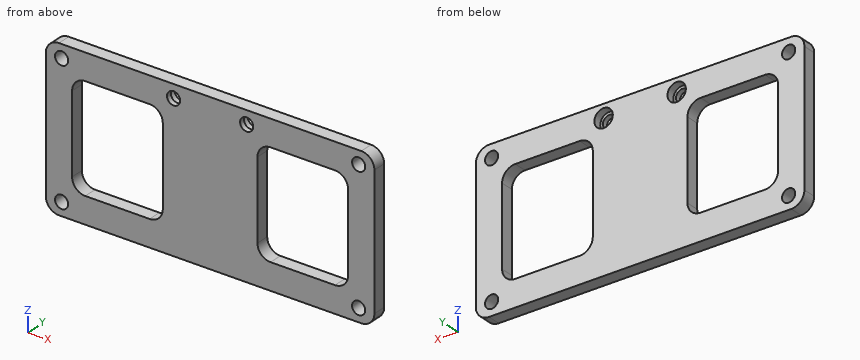
Autodesk Inventor part; units mm, degrees
ref_plane "YZ Plane" through (0, 0, 0) normal (1, 0, 0) x (0, 1, 0)
ref_plane "XZ Plane" through (0, 0, 0) normal (0, 1, 0) x (-1, 0, 0)
ref_plane "XY Plane" through (0, 0, 0) normal (0, 0, 1) x (1, 0, 0)
sketch "Sketch1" plane through (0, 0, 0) normal (0, 1, 0) x (-1, 0, 0)
  line L0 (33.3375, 19.05) -> (-33.3375, 19.05)
  line L1 (-33.3375, 19.05) -> (-33.3375, -19.05)
  line L2 (-33.3375, -19.05) -> (33.3375, -19.05)
  line L3 (33.3375, -19.05) -> (33.3375, 19.05)
  line L4 (33.3375, 19.05) -> (-33.3375, -19.05) construction
  line L5 (-33.3375, 19.05) -> (33.3375, -19.05) construction
  line L6 (39.6875, -19.05) -> (-39.6875, -19.05)
  line L7 (-39.6875, -19.05) -> (-39.6875, 19.05)
  line L8 (-39.6875, 19.05) -> (39.6875, 19.05)
  line L9 (39.6875, 19.05) -> (39.6875, -19.05)
  line L10 (39.6875, -19.05) -> (-39.6875, 19.05) construction
  line L11 (-39.6875, -19.05) -> (39.6875, 19.05) construction
  circle A0 centre (35.8775, -15.875) radius 1.5875
  circle A1 centre (35.8775, 15.875) radius 1.5875
  circle A2 centre (-35.8775, -15.875) radius 1.5875
  circle A3 centre (-35.8775, 15.875) radius 1.5875
  line L12 (33.3375, 12.7) -> (-33.3375, 12.7)
  line L13 (-33.3375, 12.7) -> (-33.3375, -12.7)
  line L14 (-33.3375, -12.7) -> (33.3375, -12.7)
  line L15 (33.3375, -12.7) -> (33.3375, 12.7)
  line L16 (11.43, 12.7) -> (-11.43, 12.7)
  line L17 (-11.43, 12.7) -> (-11.43, -12.7)
  line L18 (-11.43, -12.7) -> (11.43, -12.7)
  line L19 (11.43, -12.7) -> (11.43, 12.7)
  circle A4 centre (8.8265, 15.875) radius 1.5875
  circle A5 centre (-8.8265, 15.875) radius 1.5875
  point P0 (0, 0)
  point P1 (0, 12.7)
  point P2 (0, 0)
  point P3 (0, 0)
  point P4 (0, -12.7)
  point P5 (0, 0)
  point P6 (-11.43, -12.7)
  point P7 (-11.43, 12.7)
  point P8 (11.43, -12.7)
  point P9 (11.43, 12.7)
  dimension "d0" = 66.675
  dimension "d1" = 38.1
  dimension "d2" = 6.35
  dimension "d5" = 31.75
  dimension "d8" = 71.755
  dimension "d11" = 2.54
  dimension "d12" = 3.175
  dimension "d14" = 3.175
  dimension "d15" = 66.675
  dimension "d19" = 22.86
  dimension "d23" = 3.175
  dimension "d24" = 3.175
  dimension "d25" = 17.653
  dimension "d26" = 8.8265
  dimension "d28" = 6.35
  dimension "d29" = 6.35
extrude "Extrusion1" add sketch "Sketch1" along normal blind 3.175 contours L3 L12 L1 L0 | L8 L9 L6 L3 | L1 L6 L7 L8 | L3 L2 L1 L14 | L19 L14 L17 L12
fillet "Fillet1" radius 3.175 12 edges at (-39.6875, 1.5875, 19.05) (39.6875, 1.5875, 19.05) (-39.6875, 1.5875, -19.05) (39.6875, 1.5875, -19.05) (-33.3375, 1.5875, 12.7) (11.43, 1.5875, 12.7) (33.3375, 1.5875, 12.7) (11.43, 1.5875, -12.7) (33.3375, 1.5875, -12.7) (-11.43, 1.5875, -12.7) (-33.3375, 1.5875, -12.7) (-11.43, 1.5875, 12.7)
sketch "Sketch3" plane through (0, 3.175, 0) normal (0, 1, 0) x (1, 0, 0)
  circle A0 centre (-8.8265, -15.875) radius 1.5875
  circle A1 centre (-8.8265, -15.875) radius 2.2225
  circle A2 centre (8.8265, -15.875) radius 1.5875
  circle A3 centre (8.8265, -15.875) radius 2.2225
  point P0 (0, 0)
  dimension "d30" = 4.445
  dimension "d31" = 4.445
extrude "Extrusion2" cut sketch "Sketch3" against normal blind 1.905 contours A0 | A1 | A2 | A3
equation "\"d15\" = d0"
equation "\"d23\" = d14"
equation "\"d24\" = d14"
equation "\"d28\" = d2"
equation "\"d29\" = d2"
properties part number "Battery_Plate"
Work out the finished part from the listing and answer in its coordinate system (mm). Give positions to 0.01 mm unless a question says otherwise; leave off trailing zeros. Loops run counter-clockwise (first coordinate to the right, second up) from the corner with the lowest first, then second, coordinate; pieces in that order, holes last. Notation, with made-up numbers: (59.5, -16) -> (81.5, -16) arc R22 cw to (81.5, 8) -> close; hole circle Ø3 at (-2, -15). An arc over 180 degrees is marked (long way). Put each result on its own line as item: value. Start each with the question number.
Item 1: The part is cut by section C-C (y = 2.4). State how many separate pieces and enclosed holes the cut face has, then the cut area to 3 significant figures.
Item 2: The part is cut by section A-A (x = -16). Give the vertices of the cut face in (y, z) (3 decimals).
Item 3: Each of these flat-tipped pins is pushed along its axis until it touches: P1, Ø2.5, axis at x = 35.88, z = -15.88, coming from the +Y side; P2, Ø4, axis at x = -8.83, z = 15.88, coming from the +Y side. Where does it stop, or does it pass through?
Item 4: The part is cut by section D-D (z = -15). Give the vertices of the cut face in (x, y) (1 decimal), then the cut area to 3 significant figures.
Item 5: The part is cut by section B-B (z = -4.5). Give the vertices of the cut face in (x, y) (1 decimal).
Item 6: Find the intervals of material crossed by L1, parallel to X at y = 1.05, z = -0.5; L2, parallel to Z at x = 15, y = 2.25; L3, parallel to X at y = 2.2, z = 14, in increasing order. Write a range as [from, to].
Answers below:
1. separate pieces: 1
1. enclosed holes: 8
1. area: 1,860 mm2
2. outline: (0, -19.05) -> (3.175, -19.05) -> (3.175, -12.7) -> (0, -12.7) -> close; (0, 12.7) -> (3.175, 12.7) -> (3.175, 19.05) -> (0, 19.05) -> close
3. P1: through
3. P2: y = 1.27
4. outline: (-39.7, 0) -> (-37.2, 0) -> (-37.2, 3.2) -> (-39.7, 3.2) -> close; (-34.6, 0) -> (34.6, 0) -> (34.6, 3.2) -> (-34.6, 3.2) -> close; (37.2, 0) -> (39.7, 0) -> (39.7, 3.2) -> (37.2, 3.2) -> close
4. area: 235 mm2
5. outline: (-39.7, 0) -> (-33.3, 0) -> (-33.3, 3.2) -> (-39.7, 3.2) -> close; (-11.4, 0) -> (11.4, 0) -> (11.4, 3.2) -> (-11.4, 3.2) -> close; (33.3, 0) -> (39.7, 0) -> (39.7, 3.2) -> (33.3, 3.2) -> close
6. L1: [-39.69, -33.34], [-11.43, 11.43], [33.34, 39.69]
6. L2: [-19.05, -12.7], [12.7, 19.05]
6. L3: [-39.69, -10.02], [-7.63, 7.63], [10.02, 39.69]
